```python
from build123d import *

# Parameters (mm, degrees)
SKETCH1_W           = 80
SKETCH1_H           = 4.5
BOSS_EXTRUDE1_DEPTH = 23.6
SKETCH1_4_W         = 80
SKETCH1_4_H         = 33.5
SKETCH1_4_R         = 2
BOSS_EXTRUDE2_DEPTH = 3.6
CUT_EXTRUDE1_REACH  = 40
SKETCH2_R           = 2


with BuildPart() as part:
    # Sketch1 → Boss-Extrude1 (new body)
    with BuildSketch(Plane(origin=(0, 0, 0), x_dir=(0, 0, -1), z_dir=(1, 0, 0))):
        with Locations((0, 16.75)):
            Rectangle(SKETCH1_W, SKETCH1_H)
    extrude(amount=BOSS_EXTRUDE1_DEPTH)

    # Sketch1_4 → Boss-Extrude2 (add)
    with BuildSketch(Plane(origin=(0, 0, 0), x_dir=(0, 0, -1), z_dir=(1, 0, 0))):
        with Locations((0, -2.25)):
            Rectangle(SKETCH1_4_W, SKETCH1_4_H)
        with Locations((-35, -2)):
            Circle(SKETCH1_4_R, mode=Mode.SUBTRACT)
        with Locations((35, -2)):
            Circle(SKETCH1_4_R, mode=Mode.SUBTRACT)
    extrude(amount=BOSS_EXTRUDE2_DEPTH)

    # Sketch2 → Cut-Extrude1 (cut, up to next)
    with BuildSketch(Plane(origin=(0, 19, 0), x_dir=(1, 0, 0), z_dir=(0, 1, 0)), mode=Mode.PRIVATE) as cut_extrude1_sk1:
        with Locations((12.5, -30.950875555)):
            Circle(SKETCH2_R)
    cut_extrude1_tool1 = extrude(cut_extrude1_sk1.sketch, amount=-CUT_EXTRUDE1_REACH, mode=Mode.PRIVATE) & part.part
    add(cut_extrude1_tool1.solids().sort_by_distance((12.5, 19, 30.950876))[0], mode=Mode.SUBTRACT)
    # Sketch2 → Cut-Extrude1 (cut, up to next)
    with BuildSketch(Plane(origin=(0, 19, 0), x_dir=(1, 0, 0), z_dir=(0, 1, 0)), mode=Mode.PRIVATE) as cut_extrude1_sk2:
        with Locations((12.5, 33.54131816)):
            Circle(SKETCH2_R)
    cut_extrude1_tool2 = extrude(cut_extrude1_sk2.sketch, amount=-CUT_EXTRUDE1_REACH, mode=Mode.PRIVATE) & part.part
    add(cut_extrude1_tool2.solids().sort_by_distance((12.5, 19, -33.541318))[0], mode=Mode.SUBTRACT)


solid = part.part
```
Model file for the job. Use its own axes, mm. A direction names the side the tool comes from. Give positions to 0.01 mm unless a question says otherwise; leave off trailing zeros. Order: outer loops, then holes, each group sorted by start corner. A loop starts at its lowest first (then second) coordinate and runs counter-clockwise, first axis right, second up.
1) Mould opens along X. For faces 3 (the cylindrical face through (12.24, 16.782, 28.968)), 4 (the flat face through (3.6, -2, 1)), 5 (the flat face through (2, -19, 1)) say: +X half, -X half, draft (parallel to the pull), parting line (faces both ways), or undercut.
2) Saw through at C-C, the plane z = 35. Write the cut outline in (x, y).
3) 3-axis set-ups, long thin cutter, end or side, ignore diameter. For faces 1 (the cylindrical face through (1.775, -2.766, -36.847)), 2 (the flat face through (13, 14.5, 1)): which of +Z, -Z, +X, -X, +Y, -Y reach the whole face in a straight line?
4) Saw through at D-D, the plane z = -5. Write the cut outline in (x, y).
5) Wall check: probe 1 along X at (y, z) = (5, 32); probe 2 along Y at (x, z) = (16.75, -6.5); probe 3 along Y at (x, z) = (1.25, 35). Give the ranges that are in metal, low to high.
6) Saw through at A-A, the plane x = 12.5. Write the cut outline in (y, z).
7) Saw through at B-B, the plane y = -2. Write the cut outline in (x, z).
8) Pin check, flat tips, straight feed: pin 1 (6 mm diameter, centred on y = 10.5, z = 25, fed in from +X); pin 2 (6 mm diameter, centred on x = 14, z = -10, fed in from -Y). Stop position of each tip, or through.
Computed:
1. face 3: undercut
1. face 4: +X half
1. face 5: draft
2. outline: (0, -19) - (3.6, -19) - (3.6, -4) - (0, -4) - close; (0, 0) - (3.6, 0) - (3.6, 14.5) - (23.6, 14.5) - (23.6, 19) - (0, 19) - close
3. face 1: +X, -X
3. face 2: +Z, -Z, +X, -Y
4. outline: (0, -19) - (3.6, -19) - (3.6, 14.5) - (23.6, 14.5) - (23.6, 19) - (0, 19) - close
5. probe 1: x = 0 to 3.6
5. probe 2: y = 14.5 to 19
5. probe 3: y = -19 to -4, 0 to 19
6. outline: (14.5, -40) - (19, -40) - (19, -35.54) - (14.5, -35.54) - close; (14.5, -31.54) - (19, -31.54) - (19, 28.95) - (14.5, 28.95) - close; (14.5, 32.95) - (19, 32.95) - (19, 40) - (14.5, 40) - close
7. outline: (0, -40) - (3.6, -40) - (3.6, -37) - (0, -37) - close; (0, -33) - (3.6, -33) - (3.6, 33) - (0, 33) - close; (0, 37) - (3.6, 37) - (3.6, 40) - (0, 40) - close
8. pin 1: stops at x = 3.6
8. pin 2: stops at y = 14.5
